Check sheet for the modelled part. Datum: model origin and axes. Units: mm. Face numbers are marked on the shaded views. A direction names the side the tool comes from. Coordinates: 2 decimals unless noted, no trailing zeros. Loops run counter-clockwise (first coordinate to the right, second up) from the corner with the lowest first, then second, coordinate; pieces in that order, holes last.
```python
from build123d import *

# Parameters (mm, degrees)
F0_R     = 2.5
F1_DEPTH = 24
F0_R_2   = 11
F2_DEPTH = 2
F0_W     = 42.3
F0_H     = 42.3
F0_R_3   = 1.5
F3_DEPTH = 48
F4_R     = 5


with BuildPart() as f1:
    # F0 (on Front) → F1 (new body)
    with BuildSketch(Plane.XZ):
        Circle(F0_R)
    extrude(amount=F1_DEPTH)

    # F0 (on Front) → F2 (join)
    with BuildSketch(Plane.XZ):
        Circle(F0_R_2)
        Circle(F0_R, mode=Mode.SUBTRACT)
    extrude(amount=F2_DEPTH)

    # F0 (on Front) → F3 (join)
    with BuildSketch(Plane.XZ):
        Rectangle(F0_W, F0_H)
        with Locations((-15.5, -15.5)):
            Circle(F0_R_3, mode=Mode.SUBTRACT)
        with Locations((15.5, -15.5)):
            Circle(F0_R_3, mode=Mode.SUBTRACT)
        with Locations((-15.5, 15.5)):
            Circle(F0_R_3, mode=Mode.SUBTRACT)
        Circle(F0_R_2, mode=Mode.SUBTRACT)
        with Locations((15.5, 15.5)):
            Circle(F0_R_3, mode=Mode.SUBTRACT)
        Circle(F0_R_2)
        Circle(F0_R, mode=Mode.SUBTRACT)
        Circle(F0_R)
    extrude(amount=-F3_DEPTH)

    # F4
    f4_edges = [f1.edges().sort_by_distance(p)[0] for p in [
        (21.15, 24, 21.15),
        (21.15, 24, -21.15),
        (-21.15, 24, -21.15),
        (-21.15, 24, 21.15),
    ]]
    fillet(f4_edges, radius=F4_R)


solid = f1.part
```
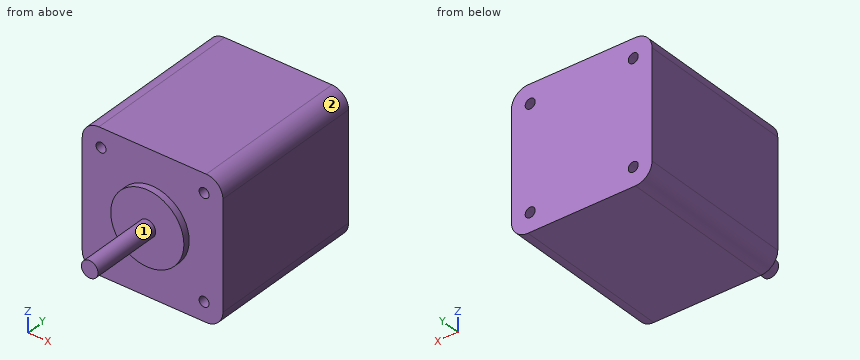
1) Section check C-C on z = 0. Enter the section's corners in (x, y).
Answer sheet:
outline: (-21.15, 0) - (-11, 0) - (-11, -2) - (-2.5, -2) - (-2.5, -24) - (2.5, -24) - (2.5, -2) - (11, -2) - (11, 0) - (21.15, 0) - (21.15, 48) - (-21.15, 48) - close
2) Section check A-A on y = 36. Enter the section's corners in (x, z).
Answer sheet:
outline: (-21.15, -16.15) arc R5 ccw to (-16.15, -21.15) - (16.15, -21.15) arc R5 ccw to (21.15, -16.15) - (21.15, 16.15) arc R5 ccw to (16.15, 21.15) - (-16.15, 21.15) arc R5 ccw to (-21.15, 16.15) - close; hole circle Ø3 at (-15.5, -15.5); hole circle Ø3 at (-15.5, 15.5); hole circle Ø3 at (15.5, -15.5); hole circle Ø3 at (15.5, 15.5)
3) Depth check by flat-ended pin: pin 1 (1.8 mm diameter, centred on x = 15.5, z = -15.5, fed in from +Y); pin 2 (1 mm diameter, centred on x = 2.5, z = -13, fed in from -Y). Enter the tip coordinate at first touch or a pass-through.
Answer sheet:
pin 1: passes through
pin 2: stops at y = 0
4) Set-up check for the marked faces 1 and 2: record each of +Z, -Z, +X, -X, +Y, -Y from which the full face is reachable in a straight line by a thin tool's end or side.
Answer sheet:
face 1: -Y
face 2: +Z, +X, +Y, -Y
5) Scan lines: line 1 (Z direction, x = 15.5, y = 11); line 2 (Z direction, x = 15, y = 10.5). Record each from-to range of solid material in increasing order.
Answer sheet:
line 1: z = -21.15 to -17, -14 to 14, 17 to 21.15
line 2: z = -21.15 to -16.91, -14.09 to 14.09, 16.91 to 21.15
6) Section check D-D on z = -10. Enter the section's corners in (x, y).
Answer sheet:
outline: (-21.15, 0) - (-4.58, 0) - (-4.58, -2) - (4.58, -2) - (4.58, 0) - (21.15, 0) - (21.15, 48) - (-21.15, 48) - close
7) Section check B-B on x = 6.5. Enter the section's corners in (y, z).
Answer sheet:
outline: (-2, -8.87) - (0, -8.87) - (0, -21.15) - (48, -21.15) - (48, 21.15) - (0, 21.15) - (0, 8.87) - (-2, 8.87) - close
